Check sheet for the modelled part. Datum: model origin and axes. Units: mm. Face numbers are marked on the shaded views. Coordinates: 2 decimals unless noted, no trailing zeros. Loops run counter-clockwise (first coordinate to the right, second up) from the corner with the lowest first, then second, coordinate; pieces in that order, holes last.
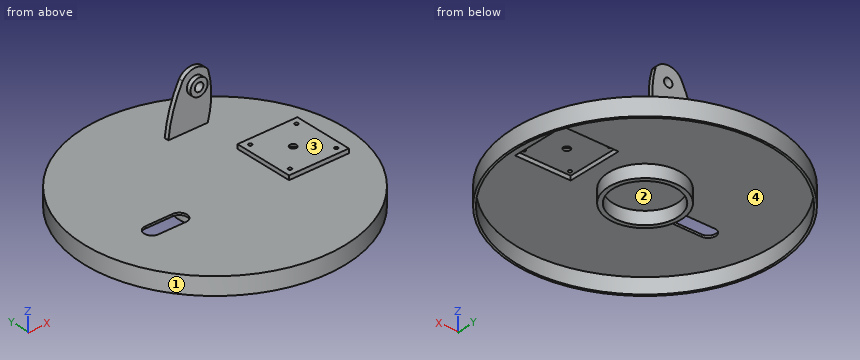
from build123d import *

# Parameters (mm, degrees)
SKETCH_1_R           = 305
EXTRUDE_1_DEPTH      = 41.2
SKETCH_2_W           = 140
SKETCH_2_H           = 140
EXTRUDE_2_DEPTH      = 10
SHELL_1_T            = -5
CUT_EXTRUDE_9_DEPTH  = 100
SKETCH_5_W           = 120
SKETCH_5_H           = 10
EXTRUDE_3_DEPTH      = 150
CUT_EXTRUDE_START    = -10
CUT_EXTRUDE_10_DEPTH = 10
SKETCH_10_R          = 10
CUT_EXTRUDE_11_DEPTH = 150
EXTRUDE_START        = 10
SKETCH_11_R          = 20
SKETCH_11_R_2        = 10
EXTRUDE_4_DEPTH      = 10
SKETCH_18_R          = 85
EXTRUDE_7_DEPTH      = 30
SKETCH_19_R          = 75
CUT_EXTRUDE_12_DEPTH = 30
SKETCH_21_R          = 4
SKETCH_21_R_2        = 8
CUT_EXTRUDE_13_DEPTH = 30


# Read off the part's stored shape, not the designer's step: the extrude step
with BuildPart() as part:
    # Sketch 1 → Extrude 1 (new body)
    with BuildSketch(Plane.XY):
        with Locations(Location((0, 0, 0), (0, 0, 180))):
            Circle(SKETCH_1_R)
    extrude(amount=EXTRUDE_1_DEPTH)

    # Sketch 2 → Extrude 2 (add)
    with BuildSketch(Plane.XY.offset(41.2)):
        with Locations((183, 0)):
            Rectangle(SKETCH_2_W, SKETCH_2_H)
    extrude(amount=EXTRUDE_2_DEPTH)

    # Shell 1
    shell_1_openings = [part.faces().sort_by_distance(p)[0] for p in [
        (0, 0, 0),
    ]]
    offset(amount=SHELL_1_T, openings=shell_1_openings, kind=Kind.INTERSECTION)

    # Sketch 4 → Cut-Extrude 9 (cut)
    with BuildSketch(Plane.XY):
        with BuildLine():
            Line((-182, -22), (-118, -22))
            ThreePointArc((-118, -22), (-100, -40), (-118, -58))
            Line((-118, -58), (-182, -58))
            ThreePointArc((-182, -58), (-200, -40), (-182, -22))
        make_face()
    extrude(amount=CUT_EXTRUDE_9_DEPTH, mode=Mode.SUBTRACT)

    # Sketch 5 → Extrude 3 (add)
    with BuildSketch(Plane.XY.offset(41.2)):
        with Locations((99, 177.019414693)):
            Rectangle(SKETCH_5_W, SKETCH_5_H)
    extrude(amount=EXTRUDE_3_DEPTH)

    # Cut-Extrude 10 outline → Cut-Extrude 10 (cut)
    with BuildSketch(Plane.XZ.offset(-172.019414693).offset(CUT_EXTRUDE_START)):
        with BuildLine():
            ThreePointArc((39, 41.2), (50.403223503, 97.919506773), (72.48168386, 151.395459716))
            ThreePointArc((72.48168386, 151.395459716), (101.995862517, 167.198851528), (131.758731658, 151.868960626))
            ThreePointArc((131.758731658, 151.868960626), (139.395350951, 96.479523786), (131, 41.2))
            Line((131, 41.2), (159, 41.2))
            Line((159, 41.2), (159, 191.2))
            Line((159, 191.2), (39, 191.2))
            Line((39, 191.2), (39, 41.2))
        make_face()
    extrude(amount=CUT_EXTRUDE_10_DEPTH, mode=Mode.SUBTRACT)

    # Sketch 10 → Cut-Extrude 11 (cut)
    with BuildSketch(Plane.XZ.offset(-172.019414693)):
        with Locations(Location((102.283418824, 131.2, 0), (0, 0, 270))):
            Circle(SKETCH_10_R)
    extrude(amount=-CUT_EXTRUDE_11_DEPTH, mode=Mode.SUBTRACT)

    # Sketch 11 → Extrude 4 (add)
    with BuildSketch(Plane.XZ.offset(-172.019414693).offset(EXTRUDE_START)):
        with Locations(Location((102.283418824, 131.2, 0), (0, 0, 90))):
            Circle(SKETCH_11_R)
        with Locations(Location((102.283418824, 131.2, 0), (0, 0, 270))):
            Circle(SKETCH_11_R_2, mode=Mode.SUBTRACT)
    extrude(amount=-EXTRUDE_4_DEPTH)

    # Sketch 18 → Extrude 7 (add)
    with BuildSketch(Plane(origin=(0, 0, 36.2), x_dir=(-1, 0, 0), z_dir=(0, 0, -1))):
        with Locations(Location((0, 0, 0), (0, 0, 180))):
            Circle(SKETCH_18_R)
    extrude(amount=EXTRUDE_7_DEPTH)

    # Sketch 19 → Cut-Extrude 12 (cut)
    with BuildSketch(Plane(origin=(0, 0, 6.2), x_dir=(-1, 0, 0), z_dir=(0, 0, -1))):
        Circle(SKETCH_19_R)
    extrude(amount=-CUT_EXTRUDE_12_DEPTH, mode=Mode.SUBTRACT)

    # Sketch 21 → Cut-Extrude 13 (cut)
    with BuildSketch(Plane.XY.offset(51.2)):
        with Locations((237, 54)):
            Circle(SKETCH_21_R)
        with Locations((129, 54)):
            Circle(SKETCH_21_R)
        with Locations((237, -54)):
            Circle(SKETCH_21_R)
        with Locations((129, -54)):
            Circle(SKETCH_21_R)
        with Locations((183, 0)):
            Circle(SKETCH_21_R_2)
    extrude(amount=-CUT_EXTRUDE_13_DEPTH, mode=Mode.SUBTRACT)


solid = part.part
(1) Draft check along Y on the marked faces 1, 2, 3 and 4. Enter one of: pulls with the +Y half, pulls with the -Y half, needs draft (parallel to the pull), parting line crosses it, or undercut.
(2) Gauge pin test, flat ends, axial feed: P1, Ø3, axis at x = -222.5, y = -177.5, coming from the -Z side; P2, Ø4, axis at x = -155.5, z = 39, coming from the -Y side; P3, Ø20, axis at x = 107, z = 127.5, coming from the -Y side; P4, Ø6.5, axis at x = 129, y = -54, coming from the +Z side. Record the tip position at first contact, or that the pin passes through.
(3) Section check D-D, the plane z = 131.2. Enter the section's corners in (x, y), plus the area to 3 significant figures.
(4) Section check B-B, the plane x = 0. Enter the section's corners in (y, z), plus the area to 3 significant figures.
(5) Section check C-C, the plane y = -40. Enter the section's corners in (x, z), plus the area to 3 significant figures.
(6) Scan lines: line 1 along Y through (x, z) = (129, 48.85); line 2 along Y through (x, z) = (0, 11); line 3 along X through (y, z) = (169, 131). Record each from-to range of solid material in increasing order.
(7) Section check A-A, the plane z = 16. Enter the section's corners in (x, y).
Determined:
1. face 1: parting line crosses it
1. face 2: undercut
1. face 3: needs draft
1. face 4: undercut
2. P1: stops at z = 36.2
2. P2: stops at y = -263.56
2. P3: stops at y = 162.02
2. P4: passes through
3. outline: (62.71, 172.02) - (82.28, 172.02) - (82.28, 162.02) - (92.28, 162.02) - (92.28, 182.02) - (62.71, 182.02) - close; (112.28, 162.02) - (122.28, 162.02) - (122.28, 172.02) - (136.52, 172.02) - (136.52, 182.02) - (112.28, 182.02) - close
3. area: 738 mm2
4. outline: (-305, 0) - (-300, 0) - (-300, 36.2) - (-85, 36.2) - (-85, 6.2) - (-75, 6.2) - (-75, 36.2) - (75, 36.2) - (75, 6.2) - (85, 6.2) - (85, 36.2) - (300, 36.2) - (300, 0) - (305, 0) - (305, 41.2) - (-305, 41.2) - close
4. area: 4,010 mm2
5. outline: (-302.37, 0) - (-297.32, 0) - (-297.32, 36.2) - (-200, 36.2) - (-200, 41.2) - (-302.37, 41.2) - close; (-100, 36.2) - (-75, 36.2) - (-75, 6.2) - (-63.44, 6.2) - (-63.44, 36.2) - (63.44, 36.2) - (63.44, 6.2) - (75, 6.2) - (75, 36.2) - (118, 36.2) - (118, 46.2) - (248, 46.2) - (248, 36.2) - (297.32, 36.2) - (297.32, 0) - (302.37, 0) - (302.37, 41.2) - (253, 41.2) - (253, 51.2) - (113, 51.2) - (113, 41.2) - (-100, 41.2) - close
5. area: 3,680 mm2
6. line 1: y = -70 to -58, -50 to 50, 58 to 70, 172.02 to 182.02
6. line 2: y = -305 to -300, -85 to -75, 75 to 85, 300 to 305
6. line 3: x = 82.28 to 92.29, 112.28 to 122.28
7. outline: circle Ø610 at (0, 0); circle Ø170 at (0, 0); hole circle Ø600 at (0, 0); hole circle Ø150 at (0, 0)
